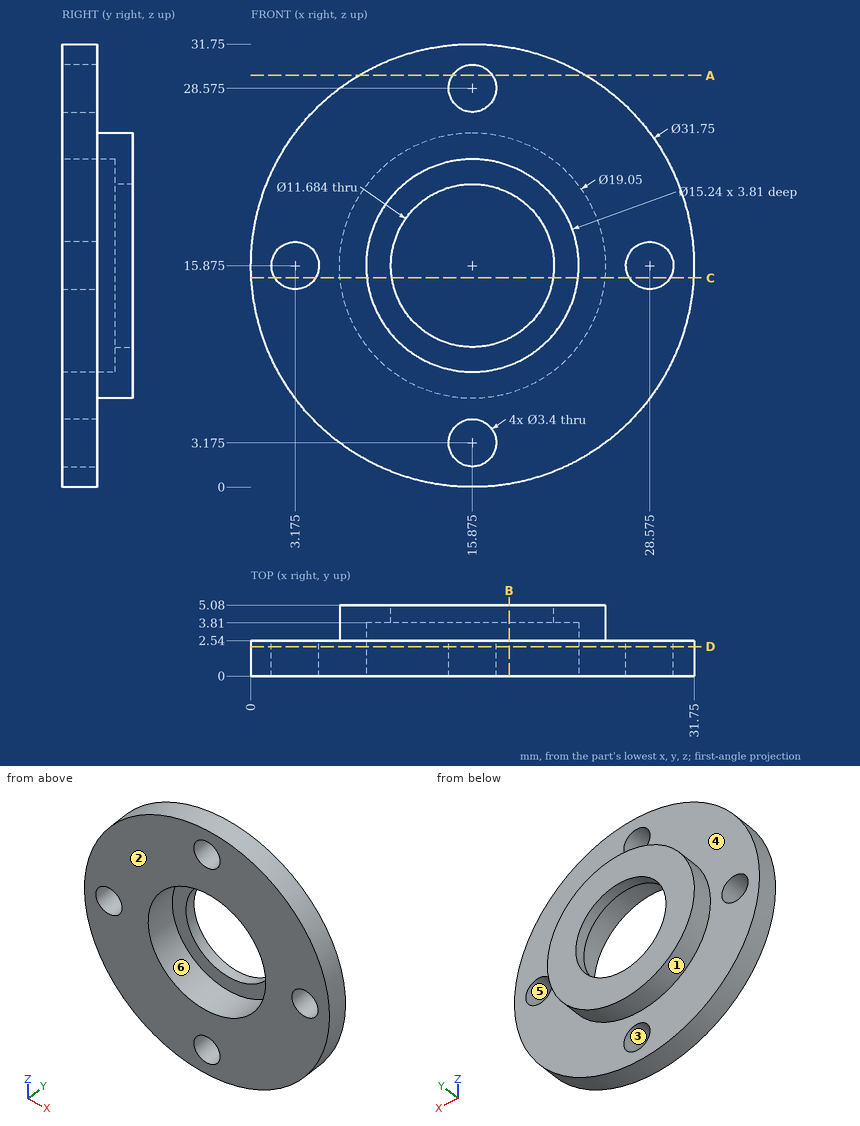
Verification items for this drawing (mm, ordinates from the low corner). A direction names the side the tool comes from. Coordinates: 2 decimals unless noted, no trailing zeros. Loops run counter-clockwise (first coordinate to the right, second up) from the corner with the lowest first, then second, coordinate; pieces in that order, holes last. Notation, with made-up numbers: (85, -10.5) - (133, -10.5) arc R21 ccw to (133, 6.5) - close; hole circle Ø6 at (24, -32.5). An arc over 180 degrees is marked (long way). One line per item, written item: value. Start each with the question number.
(1) Depth check by flat-ended pin: P1, Ø3, axis at y = 2, z = 24.5, coming from the -X side; P2, Ø8, axis at x = 3.5, z = 4.5, coming from the +Y side. Enter the tip coordinate at first touch or a pass-through.
(2) Cross-section at D-D on y = 2.1. Enter the section's corners in (x, z) (3 decimals).
(3) Mould release check, pull along Z, two halves, no side actions. Record for the marked faces 1, 2 and 3: released by +Z, released by -Z, zero draft, split by the parting line, or undercut.
(4) Cross-section at C-C on z = 15. Enter the section's corners in (x, y), plus the area to 3 significant figures.
(5) Cross-section at A-A on z = 29.5. Enter the section's corners in (x, y), plus the area to 3 significant figures.
(6) Cross-section at B-B on x = 18.5. Enter the section's corners in (y, z), plus the area to 3 significant figures.
(7) Tool access check on the marked faces 4, 5 and 6. Record the directions out of +Z, -Z, +X, -X, +Y, -Y that give a thin tool (end or side, any length) a straight path to the whole face; none if there is none.
(8) Material ranges on line 1 (Z direction, x = 2.5, y = 2.3); line 2 (Z direction, x = 16, y = 3); line 3 (X direction, y = 0.45, z = 4), recorded low to high. Write a range as [from, to].
Results below:
1. P1: stops at x = 1.69
1. P2: stops at y = 2.54
2. outline: circle Ø31.75 at (15.875, 15.875); hole circle Ø3.4 at (3.175, 15.875); hole circle Ø15.24 at (15.875, 15.875); hole circle Ø3.4 at (15.875, 3.175); hole circle Ø3.4 at (15.875, 28.575); hole circle Ø3.4 at (28.575, 15.875)
3. face 1: split by the parting line
3. face 2: zero draft
3. face 3: undercut
4. outline: (0.02, 0) - (1.72, 0) - (1.72, 2.54) - (0.02, 2.54) - close; (4.63, 0) - (8.31, 0) - (8.31, 3.81) - (10.1, 3.81) - (10.1, 5.08) - (6.39, 5.08) - (6.39, 2.54) - (4.63, 2.54) - close; (21.65, 3.81) - (23.44, 3.81) - (23.44, 0) - (27.12, 0) - (27.12, 2.54) - (25.36, 2.54) - (25.36, 5.08) - (21.65, 5.08) - close; (30.03, 0) - (31.73, 0) - (31.73, 2.54) - (30.03, 2.54) - close
4. area: 41.5 mm2
5. outline: (7.73, 0) - (14.45, 0) - (14.45, 2.54) - (7.73, 2.54) - close; (17.3, 0) - (24.02, 0) - (24.02, 2.54) - (17.3, 2.54) - close
5. area: 34.1 mm2
6. outline: (0, 0.22) - (2.54, 0.22) - (2.54, 6.72) - (5.08, 6.72) - (5.08, 10.66) - (3.81, 10.66) - (3.81, 8.72) - (0, 8.72) - close; (0, 23.03) - (3.81, 23.03) - (3.81, 21.09) - (5.08, 21.09) - (5.08, 25.03) - (2.54, 25.03) - (2.54, 31.53) - (0, 31.53) - close
6. area: 58.3 mm2
7. face 4: +Y
7. face 5: +Y, -Y
7. face 6: -Y
8. line 1: z = [7.32, 14.31], [17.44, 24.43]
8. line 2: z = [6.35, 8.26], [23.49, 25.4]
8. line 3: x = [5.34, 14.39], [17.36, 26.41]
